from build123d import *

# Parameters (mm, degrees)
SKETCH_R        = 11
PAD_DEPTH       = 8.5
SKETCH001_R     = 9.85
PAD001_DEPTH    = 2.5
SKETCH002_R     = 9
POCKET_DEPTH    = 7.5
SKETCH003_R     = 1.95
POCKET001_DEPTH = 1.5
FILLET_R        = 1.2
SKETCH005_R     = 1.1
POCKET002_DEPTH = 2
POCKET003_DEPTH = 3.5


with BuildPart() as part:
    # Sketch → Pad (new body)
    with BuildSketch(Plane.XY):
        Circle(SKETCH_R)
    extrude(amount=PAD_DEPTH)

    # Sketch001 (on Face3 of Pad) → Pad001 (join)
    with BuildSketch(Plane.XY.offset(8.5)):
        Circle(SKETCH001_R)
    extrude(amount=PAD001_DEPTH)

    # Sketch002 (on Face5 of Pad001) → Pocket (cut)
    with BuildSketch(Plane.XY.offset(11)):
        Circle(SKETCH002_R)
    extrude(amount=-POCKET_DEPTH, mode=Mode.SUBTRACT)

    # Sketch003 (on Face2 of Pocket) → Pocket001 (cut)
    with BuildSketch(Plane(origin=(0, 0, 0), x_dir=(1, 0, 0), z_dir=(0, 0, -1))):
        with Locations((0, 6.8)):
            Circle(SKETCH003_R)
        with Locations((-5.8889727457, -3.4)):
            Circle(SKETCH003_R)
        with Locations((5.8889727457, -3.4)):
            Circle(SKETCH003_R)
    extrude(amount=-POCKET001_DEPTH, mode=Mode.SUBTRACT)

    # Fillet
    fillet_edges = [part.edges().sort_by_distance(p)[0] for p in [
        (-11, 0, 0),
    ]]
    fillet(fillet_edges, radius=FILLET_R)

    # Sketch005 (on Face11 of Fillet) → Pocket002 (cut)
    with BuildSketch(Plane(origin=(0, 0, 1.5), x_dir=(1, 0, 0), z_dir=(0, 0, -1))):
        with Locations((-5.8889727457, -3.4)):
            Circle(SKETCH005_R)
        with Locations((0, 6.8)):
            Circle(SKETCH005_R)
        with Locations((5.8889727457, -3.4)):
            Circle(SKETCH005_R)
    extrude(amount=-POCKET002_DEPTH, mode=Mode.SUBTRACT)

    # Sketch007 (on Face4 of Pocket002) → Pocket003 (cut)
    with BuildSketch(Plane(origin=(0, 0, 0), x_dir=(1, 0, 0), z_dir=(0, 0, -1))):
        with BuildLine():
            ThreePointArc((-3.5353318533, 4.2132444372), (-3.3874236532, 5.9038429005), (-5.0780221165, 6.0517511006))
            ThreePointArc((-5.0780221165, 6.0517511006), (-6.8416006899, 3.95), (-7.7799812488, 1.3718206036))
            ThreePointArc((-7.7799812488, 1.3718206036), (-6.8065897584, -0.0183265132), (-5.4164426416, 0.9550649772))
            ThreePointArc((-3.5353318533, 4.2132444372), (-4.7631397208, 2.75), (-5.4164426416, 0.9550649772))
        make_face()
        with BuildLine():
            ThreePointArc((5.0780221165, 6.0517511006), (3.3874236532, 5.9038429005), (3.5353318533, 4.2132444372))
            ThreePointArc((5.4164426416, 0.9550649772), (4.7631397208, 2.75), (3.5353318533, 4.2132444372))
            ThreePointArc((5.4164426416, 0.9550649772), (6.8065897584, -0.0183265132), (7.7799812488, 1.3718206036))
            ThreePointArc((7.7799812488, 1.3718206036), (6.8416006899, 3.95), (5.0780221165, 6.0517511006))
        make_face()
        with BuildLine():
            ThreePointArc((-1.8811107883, -5.1683094143), (-3.4191661052, -5.8855163873), (-2.7019591323, -7.4235717042))
            ThreePointArc((-2.7019591323, -7.4235717042), (0, -7.9), (2.7019591323, -7.4235717042))
            ThreePointArc((2.7019591323, -7.4235717042), (3.4191661052, -5.8855163873), (1.8811107883, -5.1683094143))
            ThreePointArc((-1.8811107883, -5.1683094143), (0, -5.5), (1.8811107883, -5.1683094143))
        make_face()
        with BuildLine():
            ThreePointArc((-1.0284601755, 1.225671109), (-0.8805519754, 2.9162695724), (-2.5711504387, 3.0641777725))
            ThreePointArc((-2.5711504387, 3.0641777725), (-3.4641016151, 2), (-3.939231012, 0.6945927107))
            ThreePointArc((-3.939231012, 0.6945927107), (-2.9658395216, -0.6955544061), (-1.5756924048, 0.2778370843))
            ThreePointArc((-1.0284601755, 1.225671109), (-1.3856406461, 0.8), (-1.5756924048, 0.2778370843))
        make_face()
        with BuildLine():
            ThreePointArc((-0.5472322293, -1.5035081933), (0, -1.6), (0.5472322293, -1.5035081933))
            ThreePointArc((1.3680805733, -3.7587704831), (2.0852875463, -2.2207151662), (0.5472322293, -1.5035081933))
            ThreePointArc((-1.3680805733, -3.7587704831), (0, -4), (1.3680805733, -3.7587704831))
            ThreePointArc((-0.5472322293, -1.5035081933), (-2.0852875463, -2.2207151662), (-1.3680805733, -3.7587704831))
        make_face()
        with BuildLine():
            ThreePointArc((2.5711504387, 3.0641777725), (0.8805519754, 2.9162695724), (1.0284601755, 1.225671109))
            ThreePointArc((1.5756924048, 0.2778370843), (1.3856406461, 0.8), (1.0284601755, 1.225671109))
            ThreePointArc((1.5756924048, 0.2778370843), (2.9658395216, -0.6955544061), (3.939231012, 0.6945927107))
            ThreePointArc((3.939231012, 0.6945927107), (3.4641016151, 2), (2.5711504387, 3.0641777725))
        make_face()
    extrude(amount=-POCKET003_DEPTH, mode=Mode.SUBTRACT)


with BuildPart() as part_1:
    # Body placement: moved
    add(part.part.moved(Location((0, 1e-05, 68.2))))


solid = part_1.part
Part model, mm, in its own coordinate system. A direction names the side the tool comes from. Coordinates: 2 decimals unless noted, no trailing zeros. Loops run counter-clockwise (first coordinate to the right, second up) from the corner with the lowest first, then second, coordinate; pieces in that order, holes last. Notation, with made-up numbers: (12.5, 14.25) -> (23.5, 14.25) arc R30 ccw to (23.5, 47.25) -> close; hole circle Ø4 at (27, -34). An arc over 180 degrees is marked (long way). Use a Markdown table: item, result. Add a question column.
Item 1: Pull direction Y, two halves, no side cores. Call faces 4 (the flat face through (1, -6, 69.7)), 5 (the flat face through (3, -9, 79.2)), 6 (the cylindrical face through (-2.135, -9.616, 77.932)), 7 (the cylindrical face through (6.86, -3.92, 69.93)): +Y half, -Y half, draft (parallel to the pull), parting line (faces both ways), or undercut.
Item 2: Band-saw the part on A-A on x = 0. Give the number of separate pieces and of enclosed holes in the cut face, plus the area to 3 significant figures.
Item 3: Which spindle directions (+Z, -Z, +X, -X, +Y, -Y) get a long thin tool onto all of the face, cutting with end or side? Do faces 1 (the flat face through (-8, -6, 76.7)), 2 (the flat face through (-6, 5, 69.7)), 3 (the cylindrical face through (-6.822, -3.983, 69.926)). Say none if no direction does.
Item 4: Band-saw the part on C-C on z = 72.5. Write the cut outline in (x, y), plus the area to 3 significant figures.
Item 5: Probe probe 1 along X at (y, z) = (-7.75, 71.5); probe 2 along Y at (x, z) = (2.75, 71.25); probe 3 along X at (y, z) = (3.25, 69.25). List the from-to ranges inside material, lowest first.
Item 6: Flat gauge pins, fed straight in: P1, Ø3, axis at y = 8.5, z = 75.5, coming from the +X side; P2, Ø2, axis at y = 1.5, z = 73, coming from the -X side; P3, Ø2, axis at x = 6.5, y = 3.5, coming from the -Z side. Where does each tip first touch, or does it go through?
Geometry says:
| question | item | result |
|---|---|---|
| 1 | face 4 | undercut |
| 1 | face 5 | draft |
| 1 | face 6 | parting line |
| 1 | face 7 | undercut |
| 2 | separate pieces | 4 |
| 2 | enclosed holes | 0 |
| 2 | area | 73.6 mm² |
| 3 | face 1 | +Z |
| 3 | face 2 | -Z |
| 3 | face 3 | +Z, -Z |
| 4 | outline | circle Ø22 at (0, 0); hole circle Ø18 at (0, 0) |
| 4 | area | 126 mm² |
| 5 | probe 1 | -7.81 to -0.55, 0.55 to 7.81 |
| 5 | probe 2 | -10.65 to -2.9, 0.71 to 5.19, 7.4 to 10.65 |
| 5 | probe 3 | -10.5 to -7.83, -3.94 to -1.99, 1.99 to 3.94, 7.83 to 10.5 |
| 6 | P1 | x = 8.49 |
| 6 | P2 | x = -10.99 |
| 6 | P3 | z = 69.7 |
